Part model, mm, in its own coordinate system. A direction names the side the tool comes from. Give positions to 0.01 mm unless a question says otherwise; leave off trailing zeros. Loops run counter-clockwise (first coordinate to the right, second up) from the corner with the lowest first, then second, coordinate; pieces in that order, holes last. Notation, with made-up numbers: (-37, 31.5) -> (0, 31.5) arc R20 ccw to (0, 61.5) -> close; hole circle Ø6 at (-10, 60). An arc over 180 degrees is marked (long way). One line per question, with ' | ' between items.
```python
from build123d import *

# Parameters (mm, degrees)
SKETCH1_R            = 6.2
BOSS_EXTRUDE1_DEPTH  = 3.2
SKETCH8_R            = 6.15
BOSS_EXTRUDE5_DEPTH  = 140
SKETCH11_R           = 6.2
BOSS_EXTRUDE6_DEPTH  = 3.2
SKETCH12_R           = 3
BOSS_EXTRUDE7_DEPTH  = 140
SKETCH14_R           = 3.9
BOSS_EXTRUDE8_DEPTH  = 10
SKETCH15_R           = 6.15
BOSS_EXTRUDE9_DEPTH  = 60
SKETCH16_R           = 6.2
BOSS_EXTRUDE10_DEPTH = 94


with BuildPart() as part:
    # Sketch1 → Boss-Extrude1 (new body)
    with BuildSketch(Plane(origin=(0, 0, 0), x_dir=(1, 0, 0), z_dir=(0, 1, 0))):
        with BuildLine():
            Line((-110.589063221, 31.6), (119.210936779, 31.6))
            ThreePointArc((119.210936779, 31.6), (150.810936779, 0), (119.210936779, -31.6))
            Line((119.210936779, -31.6), (-110.589063221, -31.6))
            ThreePointArc((-110.589063221, -31.6), (-142.189063221, 0), (-110.589063221, 31.6))
        make_face()
        with Locations(Location((119.210936779, 0, 0), (0, 0, 270))):
            Circle(SKETCH1_R, mode=Mode.SUBTRACT)
    extrude(amount=BOSS_EXTRUDE1_DEPTH)

    # Sketch8 → Boss-Extrude5 (add)
    with BuildSketch(Plane(origin=(0, 3.2, 0), x_dir=(1, 0, 0), z_dir=(0, 1, 0))):
        with Locations(Location((-110.589063221, 0, 0), (0, 0, 270))):
            Circle(SKETCH8_R)
    extrude(amount=BOSS_EXTRUDE5_DEPTH)

    # Sketch11 → Boss-Extrude6 (add)
    with BuildSketch(Plane(origin=(0, 143.2, 0), x_dir=(1, 0, 0), z_dir=(0, 1, 0))):
        with BuildLine():
            Line((-110.589063221, 30.988193708), (119.210936779, 30.988193708))
            ThreePointArc((119.210936779, 30.988193708), (150.199130487, 0), (119.210936779, -30.988193708))
            Line((119.210936779, -30.988193708), (-110.589063221, -30.988193708))
            ThreePointArc((-110.589063221, -30.988193708), (-141.577256929, 0), (-110.589063221, 30.988193708))
        make_face()
        with Locations(Location((119.210936779, 0, 0), (0, 0, 270))):
            Circle(SKETCH11_R, mode=Mode.SUBTRACT)
    extrude(amount=BOSS_EXTRUDE6_DEPTH)

    # Sketch12 → Boss-Extrude7 (add)
    with BuildSketch(Plane(origin=(0, 3.2, 0), x_dir=(1, 0, 0), z_dir=(0, 1, 0))):
        with Locations(Location((-43.639063221, 0, 0), (0, 0, 270))):
            Circle(SKETCH12_R)
    extrude(amount=BOSS_EXTRUDE7_DEPTH)

    # Sketch14 → Boss-Extrude8 (add)
    with BuildSketch(Plane(origin=(0, 3.2, 0), x_dir=(1, 0, 0), z_dir=(0, 1, 0))):
        with Locations(Location((53.310936779, 0, 0), (0, 0, 270))):
            Circle(SKETCH14_R)
    boss_extrude8 = extrude(amount=BOSS_EXTRUDE8_DEPTH)

    # Sketch15 → Boss-Extrude9 (add)
    with BuildSketch(Plane(origin=(0, 13.2, 0), x_dir=(1, 0, 0), z_dir=(0, 1, 0))):
        with Locations(Location((53.310936779, 0, 0), (0, 0, 270))):
            Circle(SKETCH15_R)
    boss_extrude9 = extrude(amount=BOSS_EXTRUDE9_DEPTH)

    # Mirror7: Boss-Extrude8, Boss-Extrude9 across plane
    add(boss_extrude8.mirror(Plane.ZX.offset(73.2)))
    add(boss_extrude9.mirror(Plane.ZX.offset(73.2)))

    # Sketch16 → Boss-Extrude10 (add, symmetric)
    with BuildSketch(Plane(origin=(0, 73.2, 0), x_dir=(-1, 0, 0), z_dir=(0, -1, 0))):
        with Locations(Location((110.589063221, 0, 0), (0, 0, 270))):
            Circle(SKETCH16_R)
    extrude(amount=BOSS_EXTRUDE10_DEPTH, both=True)


solid = part.part
```
1) Drill centre lines: line 1 (X direction, y = 55, z = 0.5); line 2 (X direction, y = 1.9, z = 0); line 3 (Y direction, x = 31, z = -22). Where is each one in solid material? Low to high.
Found:
line 1: -116.77 to -104.41, -46.6 to -40.68, 47.18 to 59.44 | line 2: -142.19 to 113.01, 125.41 to 150.81 | line 3: 0 to 3.2, 143.2 to 146.4
2) Saw through at B-B (z = -16.5). Give the cut face in (x, y), and give its area (3 significant figures).
Found:
outline: (-137.54, 0) -> (146.16, 0) -> (146.16, 3.2) -> (-137.54, 3.2) -> close; (-136.82, 143.2) -> (145.44, 143.2) -> (145.44, 146.4) -> (-136.82, 146.4) -> close | area: 1,810 mm2
3) Tool access for faces 1 (the cylindrical face through (-116.736, -10.546, -0.807)), 2 (the cylindrical face through (-116.736, 72.22, -0.807)), 3 (the cylindrical face through (-116.736, 156.654, -0.807)), 4 (the cylindrical face through (150.19, 144.78, -0.68)): list every direction of +Z, -Z, +X, -X, +Y, -Y with a clear straight run to the whole face (end or side of a thin tool).
Found:
face 1: -Y | face 2: none | face 3: +Y | face 4: +X, +Y
4) Saw through at A-A (x = -83.5). Give the cut face in (y, z), and give its area (3 significant figures).
Found:
outline: (0, -31.6) -> (3.2, -31.6) -> (3.2, 31.6) -> (0, 31.6) -> close; (143.2, -30.99) -> (146.4, -30.99) -> (146.4, 30.99) -> (143.2, 30.99) -> close | area: 401 mm2
5) Pull direction Z, two halves, no side cores. Call faces 5 (the flat face through (49, 133.2, 0)), 6 (the cylindrical face through (-142.18, 1.58, 0.69)), 7 (the cylindrical face through (125.358, 144.778, -0.807)): pulls with the +Z half, pulls with the -Z half, needs draft (parallel to the pull), parting line crosses it, or undercut.
Found:
face 5: needs draft | face 6: parting line crosses it | face 7: undercut
6) Saw through at C-C (y = 86). Give the cut face in (x, z).
Found:
outline: circle Ø12.4 at (-110.59, 0); circle Ø6 at (-43.64, 0); circle Ø12.3 at (53.31, 0)
7) Pin check, flat tips, straight feed: P1, Ø10, axis at x = -63.5, z = 23, coming from the +Y side; P2, Ø12, axis at y = 102, z = -10, coming from the -X side; P3, Ø3, axis at x = -58, z = -16, coming from the -Y side. Stop position of each tip, or through.
Found:
P1: y = 146.4 | P2: x = -115.33 | P3: y = 0
8) Saw through at D-D (z = 0). State how many separate pieces and enclosed holes the cut face has, and give its area (3 significant figures).
Found:
separate pieces: 3 | enclosed holes: 2 | area: 6,520 mm2
